Part model, mm, in its own coordinate system. Face numbers are marked on the shaded views. A direction names the side the tool comes from. Round coordinates to 2 decimals unless told otherwise and drop trailing zeros. Loops run counter-clockwise (first coordinate to the right, second up) from the corner with the lowest first, then second, coordinate; pieces in that order, holes last.
1) Drop flat-ended pins along their axis: P1, Ø5, axis at x = 10, z = 16, coming from the +Y side; P2, Ø13.5, axis at x = 22.5, z = 25.5, coming from the +Y side; P3, Ø12, axis at x = 15.5, z = 34.5, coming from the +Y side. Give the stop position or say it passes through.
2) 3-axis set-ups, long thin cutter, end or side, ignore diameter. For the marked faces 1 and 2: which of +Z, -Z, +X, -X, +Y, -Y reach the whole face in a straight line?
3) Band-saw the part on B-B, the plane x = 24. Write the cut outline in (y, z), then the cut area to 3 significant figures.
4) Mould opens along X. For the marked faces 3, 4, 5 and 6 say: +X half, -X half, draft (parallel to the pull), parting line (faces both ways), or undercut.
5) Band-saw the part on D-D, the plane x = 34.5. Write the cut outline in (y, z).
6) Probe line 1 (X direction, y = 12, z = 20.5); line 2 (X direction, y = 29, z = 21); line 3 (Y direction, x = 12, z = 15.5). List the from-to ranges inside material, lowest first.
7) Band-saw the part on A-A, the plane z = 21. Write the cut outline in (x, y).
8) Band-saw the part on C-C, the plane y = 29. Write the cut outline in (x, z).
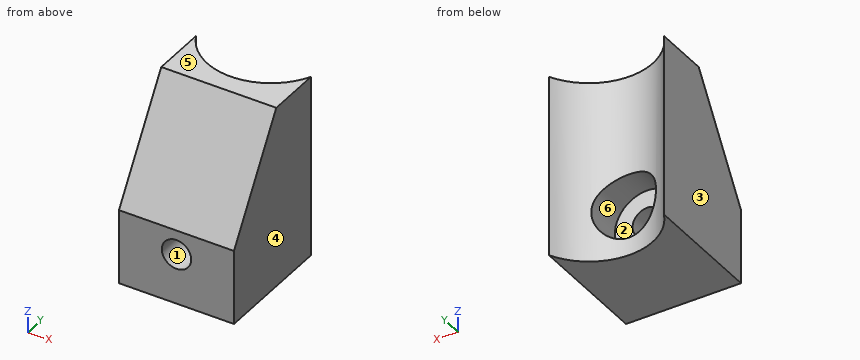
from build123d import *

# Parameters (mm, degrees)
BOSS_EXTRUDE1_DEPTH = 76.2
CUT_EXTRUDE1_DEPTH  = 49.2
SKETCH5_R           = 6.15
CUT_EXTRUDE2_DEPTH  = 44
SKETCH6_R           = 13.5
CUT_EXTRUDE3_DEPTH  = 27


with BuildPart() as part:
    # Sketch2 → Boss-Extrude1 (new body)
    with BuildSketch(Plane.XY):
        with BuildLine():
            Line((0, 51), (0, 0))
            Line((0, 0), (48, 0))
            Line((48, 0), (48, 51))
            ThreePointArc((48, 51), (24, 35.983160819), (0, 51))
        make_face()
    extrude(amount=BOSS_EXTRUDE1_DEPTH)

    # Sketch3 → Cut-Extrude1 (cut)
    with BuildSketch(Plane.ZY.offset(-48)):
        Polygon((76.2, 28), (76.2, 0), (31.2, 0), align=None)
    extrude(amount=CUT_EXTRUDE1_DEPTH, mode=Mode.SUBTRACT)

    # Sketch5 → Cut-Extrude2 (cut)
    with BuildSketch(Plane.XZ):
        with Locations((24, 21)):
            Circle(SKETCH5_R)
    extrude(amount=-CUT_EXTRUDE2_DEPTH, mode=Mode.SUBTRACT)

    # Sketch6 → Cut-Extrude3 (cut)
    with BuildSketch(Plane(origin=(0, 51, 0), x_dir=(-1, 0, 0), z_dir=(0, -1, 0))):
        with Locations((-24, -21)):
            Circle(SKETCH6_R)
    extrude(amount=CUT_EXTRUDE3_DEPTH, mode=Mode.SUBTRACT)


solid = part.part
Reported:
1. P1: stops at y = 41.7
1. P2: stops at y = 24
1. P3: stops at y = 40.27
2. face 1: +Y, -Y
2. face 2: +Y
3. outline: (0, 0) - (35.98, 0) - (35.98, 7.5) - (24, 7.5) - (24, 14.85) - (0, 14.85) - close; (0, 27.15) - (24, 27.15) - (24, 34.5) - (35.98, 34.5) - (35.98, 76.2) - (28, 76.2) - (0, 31.2) - close
3. area: 1,490 mm2
4. face 3: -X half
4. face 4: +X half
4. face 5: draft
4. face 6: undercut
5. outline: (0, 0) - (38.14, 0) - (38.14, 12.51) - (24, 12.51) - (24, 29.49) - (38.14, 29.49) - (38.14, 76.2) - (28, 76.2) - (0, 31.2) - close
6. line 1: x = 0 to 17.87, 30.13 to 48
6. line 2: x = 0 to 10.5, 37.5 to 48
6. line 3: y = 0 to 24
7. outline: (0, 0) - (17.85, 0) - (17.85, 24) - (10.5, 24) - (10.5, 39.65) arc R26.69 cw to (0, 51) - close; (30.15, 0) - (48, 0) - (48, 51) arc R26.69 cw to (37.5, 39.65) - (37.5, 24) - (30.15, 24) - close
8. outline: (0, 0) - (48, 0) - (48, 76.2) - (0, 76.2) - close; hole circle Ø27 at (24, 21)
